The model under review builds one solid part; all positions refer to its coordinate system, in mm. Face numbers are marked on the shaded views. A direction names the side the tool comes from. Round coordinates to 2 decimals unless told otherwise and drop trailing zeros. Loops run counter-clockwise (first coordinate to the right, second up) from the corner with the lowest first, then second, coordinate; pieces in that order, holes last. Notation, with made-up numbers: M 29,53 L 37,53 A29 cw 37,84 Z; hole C 57.5,-35 d9. An arc over 180 degrees is marked long. Use a Markdown table: item, result. Add a question column.
```python
from build123d import *

# Parameters (mm, degrees)
SKETCH1_W                 = 24.25
SKETCH1_H                 = 20
EXTRUDE1_DEPTH            = 54.7
CUT_EXTRUDE1_DEPTH        = 21
SKETCH5_W                 = 12.7
SKETCH5_H                 = 20
EXTRUDE2_DEPTH            = 15.1
F_8_CLEARANCE_HOLE1_D     = 4.4958
F_4_40_TAPPED_HOLE1_D     = 2.2606
F_4_40_TAPPED_HOLE1_DEPTH = 8.8646
F_4_40_TAPPED_HOLE1_TIP   = 0.679152758
SKETCH11_W                = 12.7
SKETCH11_H                = 20
CUT_EXTRUDE2_DEPTH        = 5.08
FILLET1_R                 = 1.27
SKETCH12_W                = 0.25
SKETCH12_H                = 20
CUT_EXTRUDE3_DEPTH        = 0.25
EXTRUDE3_DEPTH            = 3.175
SKETCH14_W                = 6.35
SKETCH14_H                = 0.25
CUT_EXTRUDE4_DEPTH        = 0.25


with BuildPart() as part:
    # Sketch1 → Extrude1 (new body)
    with BuildSketch(Plane.XY):
        with Locations((12.125, 0)):
            Rectangle(SKETCH1_W, SKETCH1_H)
    extrude(amount=EXTRUDE1_DEPTH)

    # Sketch4 → Cut-Extrude1 (cut, through all)
    with BuildSketch(Plane.XZ.offset(10)):
        with BuildLine():
            Line((0, 12.7), (3.95, 12.7))
            ThreePointArc((3.95, 12.7), (8.440128061, 14.559871939), (10.3, 19.05))
            Line((10.3, 19.05), (10.3, 54.7))
            Line((10.3, 54.7), (0, 54.7))
            Line((0, 54.7), (0, 12.7))
        make_face()
    extrude(amount=-CUT_EXTRUDE1_DEPTH, mode=Mode.SUBTRACT)

    # Sketch5 → Extrude2 (add)
    with BuildSketch(Plane.ZY):
        with Locations((6.35, 0)):
            Rectangle(SKETCH5_W, SKETCH5_H)
    extrude(amount=EXTRUDE2_DEPTH)

    # #8 Clearance Hole1 (through all)
    with Locations(Plane(origin=(24.25, 0, 0), x_dir=(0, 0, -1), z_dir=(1, 0, 0))):
        with Locations((-6.35, 4.7625), (-6.35, -4.7625)):
            Hole(F_8_CLEARANCE_HOLE1_D / 2)

    # #4-40 Tapped Hole1
    with Locations(Plane.XY.offset(54.7)):
        with Locations((17.9, 0)):
            Hole(F_4_40_TAPPED_HOLE1_D / 2, depth=F_4_40_TAPPED_HOLE1_DEPTH)
            with Locations((0, 0, -(F_4_40_TAPPED_HOLE1_DEPTH + F_4_40_TAPPED_HOLE1_TIP / 2))):  # 118° drill point
                Cone(0, F_4_40_TAPPED_HOLE1_D / 2, F_4_40_TAPPED_HOLE1_TIP, mode=Mode.SUBTRACT)

    # Sketch11 → Cut-Extrude2 (cut)
    with BuildSketch(Plane(origin=(24.25, 0, 0), x_dir=(0, 0, -1), z_dir=(1, 0, 0))):
        with Locations((-6.35, 0)):
            Rectangle(SKETCH11_W, SKETCH11_H)
    extrude(amount=-CUT_EXTRUDE2_DEPTH, mode=Mode.SUBTRACT)

    # Fillet1
    fillet1_edges = [part.edges().sort_by_distance(p)[0] for p in [
        (19.17, 0, 12.7),
    ]]
    fillet(fillet1_edges, radius=FILLET1_R)

    # Sketch12 → Cut-Extrude3 (cut)
    with BuildSketch(Plane(origin=(19.17, 0, 0), x_dir=(0, 0, -1), z_dir=(1, 0, 0))):
        with Locations((-6.35, 0)):
            Rectangle(SKETCH12_W, SKETCH12_H)
    extrude(amount=-CUT_EXTRUDE3_DEPTH, mode=Mode.SUBTRACT)

    # Sketch13 → Extrude3 (add, symmetric)
    with BuildSketch(Plane(origin=(0, 0, 0), x_dir=(1, 0, 0), z_dir=(0, 1, 0))):
        Polygon((-15.1, -12.7), (10.3, -54.7), (10.3, -12.7), align=None)
    extrude(amount=EXTRUDE3_DEPTH, both=True)

    # Sketch14 → Cut-Extrude4 (cut)
    with BuildSketch(Plane.XY.offset(54.7)):
        with Locations((21.075, 0)):
            Rectangle(SKETCH14_W, SKETCH14_H)
    extrude(amount=-CUT_EXTRUDE4_DEPTH, mode=Mode.SUBTRACT)


solid = part.part
```
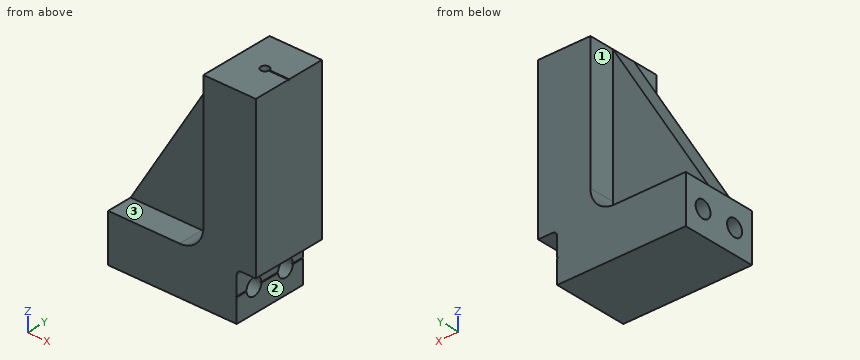
(1) To check wall thickness, follow probe 1 along Y at (x, z) = (-3.5, 6.35); probe 2 along Z at (x, y) = (11, 5); probe 3 along Y at (x, z) = (-2.5, 27) (3 decimals). State the ranges of each line that lie inside material, in increasing order.
(2) Consider section B-B, the plane y = 3.75. Give the boundary of the cut face in (x, z).
(3) Insertion check: pin 1 Ø8 at (x, z) = (2.5, 22) entering from -Y (3 decimals); pin 2 Ø1.1 at (x, y) = (22.5, 0.5) entering from -Z; pin 3 Ø5.5 at (x, y) = (-6, 7.5) entering from +Z. Each pin has a flat end and moves straight along its axis. Give the tip position at first contact, or say it passes through.
(4) Consider section A-A, the plane x = 9. Give the number of separate pieces and of enclosed holes in the cut face, then the cut area to 3 significant figures.
(5) For the marked faces 1, 2 and 3, list the 3-axis set-ups (+Z, -Z, +X, -X, +Y, -Y) from which the entire face can be reached by the end or side of a thin tool; tool diameter is ignored.
(6) Consider section C-C, the plane z = 20. Give the boundary of the cut face in (x, y) (3 decimals).
Found:
| question | item | result |
|---|---|---|
| 1 | probe 1 | y = -10 to -7.01, -2.51 to 2.51, 7.01 to 10 |
| 1 | probe 2 | z = 0 to 4.11, 8.59 to 54.7 |
| 1 | probe 3 | y = -3.175 to 3.175 |
| 2 | outline | M -15.1,0 L 19.17,0 L 19.17,4.34 L -15.1,4.34 Z; M -15.1,8.36 L 19.17,8.36 L 19.17,11.43 A1.27 cw 20.44,12.7 L 24.25,12.7 L 24.25,54.7 L 10.3,54.7 L 10.3,19.05 A6.35 cw 3.95,12.7 L -15.1,12.7 Z |
| 3 | pin 1 | stops at y = -3.175 |
| 3 | pin 2 | stops at z = 12.7 |
| 3 | pin 3 | stops at z = 12.7 |
| 4 | separate pieces | 1 |
| 4 | enclosed holes | 2 |
| 4 | area | 509 mm^2 |
| 5 | face 1 | +Z, -X, +Y |
| 5 | face 2 | -Z, +X, +Y, -Y |
| 5 | face 3 | +Z, -X, -Y |
| 6 | outline | M -10.685,-3.175 L 10.3,-3.175 L 10.3,-10 L 24.25,-10 L 24.25,10 L 10.3,10 L 10.3,3.175 L -10.685,3.175 Z |
